Design review of the part built by this model. Coordinates are the model's own, in mm. Coordinates: 2 decimals unless noted, no trailing zeros. Loops run counter-clockwise (first coordinate to the right, second up) from the corner with the lowest first, then second, coordinate; pieces in that order, holes last. Notation, with made-up numbers: (53, 42) -> (110, 42) arc R29 ccw to (110, 75) -> close; hole circle Ø5 at (-31, -25.5). An arc over 180 degrees is marked (long way). Use one line per item in the form item = value. Start each with the question number.
1. Consider section A-A (x = -5). State the section outline as (y, z) points, then the cut area to 3 significant figures.
2. Consider section B-B (y = -5.5). State the section outline as (x, z) points.
3. For pin 1 (8 mm diameter, centred on y = -8.5, z = -0.5, fed in from +X); pin 2 (6 mm diameter, centred on y = -3, z = -9.5, fed in from -X); pin 3 (6 mm diameter, centred on y = -3.5, z = -24.5, fed in from -X), all flat-tipped, find the tip position at first contact; note any pin that passes through.
4. The part is to be moulded in two halves that separate along X. For faces 1 (the face through (-17.11, -21.97, 7.77)), 2 (the face through (-17.11, -21.97, -18.23)), 3 (the face through (12, -24, -18)), 4 (the face through (12.845, -21.972, -17.971)), say which applies: released by +X, released by -X, zero draft, split by the parting line, or undercut.
5. Wall thickness on line 1 (Y direction, x = -38, z = -4.5); line 2 (X direction, y = -10.75, z = -3); line 3 (X direction, y = -17.5, z = -1.5): over which ranges is each line inside the solid? List them lowest first. Write a range as from..to.
from build123d import *

# Parameters (mm, degrees)
F1_DEPTH = 20
F2_R     = 1
F3_DEPTH = 4


with BuildPart() as f1:
    # F0 (on Front) → F1 (new body)
    with BuildSketch(Plane.XZ):
        Polygon((30, 32.439652), (0, 32.439652), (-30, 32.439652), (-55, -38.271026), (0, -38.271026), (55, -38.271026), align=None)
    extrude(amount=F1_DEPTH)

    # F2 (on face) → F3 (join)
    with BuildSketch(Plane.XZ.offset(20)):
        with Locations((-16.109127, 7.728974)):
            Circle(F2_R)
        with Locations((-16.109127, -18.271026)):
            Circle(F2_R)
        with Locations((11.890873, -18.271026)):
            Circle(F2_R)
    extrude(amount=F3_DEPTH)


solid = f1.part
Geometry check:
q1.outline = (-20, -38.27) -> (0, -38.27) -> (0, 32.44) -> (-20, 32.44) -> close
q1.area = 1,410 mm²
q2.outline = (-55, -38.27) -> (55, -38.27) -> (30, 32.44) -> (-30, 32.44) -> close
q3.pin_1 = 43.06
q3.pin_2 = -45.89
q3.pin_3 = -51.19
q4.face_1 = split by the parting line
q4.face_2 = undercut
q4.face_3 = zero draft
q4.face_4 = undercut
q5.line_1 = -20..0
q5.line_2 = -42.53..42.53
q5.line_3 = -42..42
